CAD build for the part. Positions are in the model's coordinates, mm. A direction names the side the tool comes from. Coordinates: 2 decimals unless noted, no trailing zeros. Loops run counter-clockwise (first coordinate to the right, second up) from the corner with the lowest first, then second, coordinate; pieces in that order, holes last. Notation, with made-up numbers: (76, -18) -> (118, -18) arc R16 cw to (118, 6) -> close; hole circle Ø1 at (80, 66). An arc over 180 degrees is marked (long way). Write item = value, one per line. Start each with the question number.
(1) Band-saw the part on D-D (x = 70.5). Write the cut outline in (y, z), and give its area (3 significant figures).
(2) Band-saw the part on C-C (y = 94). Write the cut outline in (x, z).
(3) Tool access for faces 4 (the face through (44, 72, 19.05)), 5 (the face through (25.4, 127, 10)), 6 (the face through (82.64, 37.83, 9.66)): list every direction of +Z, -Z, +X, -X, +Y, -Y with a clear straight run to the whole face (end or side of a thin tool).
(4) Band-saw the part on B-B (z = 3.5). Write the cut outline in (x, y), and give its area (3 significant figures).
(5) Flat gauge pins, fed straight in: P1, Ø4, axis at x = 56, y = 45.5, coming from the +Z side; P2, Ø5, axis at x = 13.5, z = 35, coming from the +Y side. Where does each tip first touch, or does it go through?
(6) Band-saw the part on A-A (x = 6.5). Write the cut outline in (y, z).
(7) Pull direction Y, two halves, no side cores. Call faces 1 (the face through (0, 10, 22)), 2 (the face through (76, 152.4, 9)), 3 (the face through (82, 57.15, 10)): +Y half, -Y half, draft (parallel to the pull), parting line (faces both ways), or undercut.
(8) Drill centre lines: line 1 (Z direction, x = 11, y = 51); line 2 (X direction, y = 95, z = 15.5). Where is each one in solid material? Low to high. Write a range as from..to.
Autodesk Inventor part; units mm, degrees
ref_plane "YZ Plane" through (0, 0, 0) normal (1, 0, 0) x (0, 1, 0)
ref_plane "XZ Plane" through (0, 0, 0) normal (0, 1, 0) x (-1, 0, 0)
ref_plane "XY Plane" through (0, 0, 0) normal (0, 0, 1) x (1, 0, 0)
sketch "Sketch1" plane through (0, 0, 0) normal (0, 0, 1) x (1, 0, 0)
  line L0 (0, 0) -> (88.9, 0)
  line L1 (88.9, 0) -> (88.9, 152.4)
  line L2 (88.9, 152.4) -> (0, 152.4)
  line L3 (0, 152.4) -> (0, 0)
  dimension "d0" = 152.4
  dimension "d1" = 88.9
extrude "Extrusion1" add sketch "Sketch1" along normal blind 19.05
sketch "Sketch2" plane through (0, 0, 19.05) normal (0, 0, 1) x (1, 0, 0)
  line L0 (0, 0) -> (88.9, 0)
  line L1 (88.9, 0) -> (88.9, 19.05)
  line L2 (88.9, 19.05) -> (0, 19.05)
  line L3 (0, 19.05) -> (0, 0)
  line L4 (88.9, 0) -> (88.9, 152.4)
  dimension "d4" = 19.05
extrude "Extrusion2" add sketch "Sketch2" along normal blind 25.4
sketch "Sketch3" plane through (0, 0, 19.05) normal (0, 0, 1) x (1, 0, 0)
  line L0 (25.4, 166.2997) -> (63.5, 166.2997)
  line L1 (63.5, 166.2997) -> (63.5, 101.6)
  line L2 (63.5, 101.6) -> (25.4, 101.6)
  line L3 (25.4, 101.6) -> (25.4, 166.2997)
  line L4 (88.9, 152.4) -> (0, 152.4)
  arc A0 (25.6076, 101.6) -> (63.2924, 101.6) centre (44.45, 101.6) ccw
  point P0 (0, 0)
  dimension "d7" = 25.4
  dimension "d8" = 25.4
  dimension "d9" = 50.8
extrude "Extrusion3" cut sketch "Sketch3" against normal blind 25.4
sketch "Sketch4" plane through (0, 0, 19.05) normal (0, 0, 1) x (1, 0, 0)
  line L0 (0, 19.05) -> (12.7, 57.15)
  line L1 (12.7, 57.15) -> (0, 57.15)
  line L2 (0, 19.05) -> (88.9, 19.05)
  line L3 (0, 19.05) -> (0, 57.15)
  line L4 (0, 152.4) -> (0, 0)
  line L5 (88.9, 19.05) -> (88.9, 57.15)
  line L6 (88.9, 0) -> (88.9, 152.4)
  line L7 (76.2, 57.15) -> (88.9, 19.05)
  line L8 (76.2, 57.15) -> (88.9, 57.15)
  line L9 (88.9, 19.05) -> (88.9, 57.15)
  dimension "d12" = 12.7
  dimension "d13" = 38.1
  dimension "d14" = 12.7
  dimension "d15" = 38.1
extrude "Extrusion4" cut sketch "Sketch4" against normal blind 25.4 contours L3 L1 L0
sketch "Sketch5" plane through (0, 0, 19.05) normal (0, 0, 1) x (1, 0, 0)
  line L0 (88.9, 19.05) -> (76.2, 57.15)
  line L1 (76.2, 57.15) -> (88.9, 57.15)
  line L2 (88.9, 19.05) -> (88.9, 152.4)
  point P0 (0, 0)
  dimension "d18" = 12.7
  dimension "d19" = 38.1
extrude "Extrusion5" cut sketch "Sketch5" against normal blind 25.4
properties part number "Guide Fork CAD" material "Aluminum 6061"
Findings below:
q1.outline = (0, 0) -> (152.4, 0) -> (152.4, 19.05) -> (19.05, 19.05) -> (19.05, 44.45) -> (0, 44.45) -> close
q1.area = 3,390 mm²
q2.outline = (0, 0) -> (27.21, 0) -> (27.21, 19.05) -> (0, 19.05) -> close; (61.69, 0) -> (88.9, 0) -> (88.9, 19.05) -> (61.69, 19.05) -> close
q3.face_4 = +Z, +X, -X, +Y
q3.face_5 = +Z, -Z, +Y
q3.face_6 = +Z, -Z, +X
q4.outline = (0, 0) -> (88.9, 0) -> (88.9, 19.05) -> (76.2, 57.15) -> (88.9, 57.15) -> (88.9, 152.4) -> (63.5, 152.4) -> (63.5, 101.6) -> (63.29, 101.6) arc R18.84 cw to (25.61, 101.6) -> (25.4, 101.6) -> (25.4, 152.4) -> (0, 152.4) -> (0, 57.15) -> (12.7, 57.15) -> (0, 19.05) -> close
q4.area = 10,600 mm²
q5.P1 = 19.05
q5.P2 = 19.05
q6.outline = (0, 0) -> (38.55, 0) -> (38.55, 19.05) -> (19.05, 19.05) -> (19.05, 44.45) -> (0, 44.45) -> close; (57.15, 0) -> (152.4, 0) -> (152.4, 19.05) -> (57.15, 19.05) -> close
q7.face_1 = draft
q7.face_2 = +Y half
q7.face_3 = undercut
q8.line_1 = 0..19.05
q8.line_2 = 0..26.8, 62.1..88.9
